Check sheet for the modelled part. Datum: model origin and axes. Units: mm. Face numbers are marked on the shaded views. Coordinates: 2 decimals unless noted, no trailing zeros. Write each loop counter-clockwise with the first axis right and the second up, starting at its lowest first coordinate (ties: lowest second). Pieces come first, ordered by that corner, then holes. Notation, with made-up numbers: (-12, 18.5) - (-5, 18.5) arc R22 cw to (-5, 25.5) - close; hole circle Ø8 at (74.25, 71). An arc over 180 degrees is marked (long way). Use one line per item in the form item = value. Start each with the question number.
1. Draft check along X on the marked faces 1, 2, 3 and 4. Enter one of: +X half, -X half, draft (parallel to the pull), parting line (faces both ways), or undercut.
2. Cross-section at A-A on x = 0. Record the boundary of the cut face in (y, z).
3. Cross-section at C-C on y = 0.75. Record the boundary of the cut face in (x, z).
4. Go/stop test with flat-tipped pins: pin 1 Ø5 at (y, z) = (1, 17) entering from +X; pin 2 Ø2 at (x, y) = (0.5, -1) entering from +Z; pin 3 Ø5.5 at (x, y) = (0, 0) entering from -Z. Record where each tip stops, or that it passes through.
5. Cross-section at B-B on z = -17. Record the boundary of the cut face in (x, y).
6. Scan lines: line 1 along Y through (x, z) = (0, 26.5); line 2 along X through (y, z) = (0, 29.25); line 3 along X through (y, z) = (0, 23.35). Record each from-to range of solid material in increasing order.
7. Cross-section at D-D on y = -5.25. Record the boundary of the cut face in (x, z).
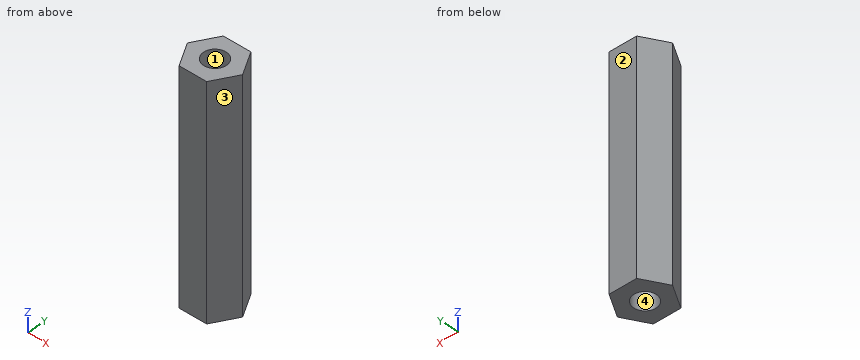
Autodesk Inventor part; units mm, degrees
ref_plane "YZ Plane" through (0, 0, 0) normal (1, 0, 0) x (0, 1, 0)
ref_plane "XZ Plane" through (0, 0, 0) normal (0, 1, 0) x (-1, 0, 0)
ref_plane "XY Plane" through (0, 0, 0) normal (0, 0, 1) x (1, 0, 0)
sketch "Sketch1" plane through (0, 0, 0) normal (0, 0, 1) x (1, 0, 0)
  line L0 (3.6662, 6.35) -> (7.3323, 0)
  line L1 (7.3323, 0) -> (3.6662, -6.35)
  line L2 (3.6662, -6.35) -> (-3.6662, -6.35)
  line L3 (-3.6662, -6.35) -> (-7.3323, 0)
  line L4 (-7.3323, 0) -> (-3.6662, 6.35)
  line L5 (-3.6662, 6.35) -> (3.6662, 6.35)
  circle A0 centre (0, 0) radius 2.0193
  dimension "d0" = 12.7
  dimension "d3" = 4.0386
extrude "Extrusion2" add sketch "Sketch1" along normal mid plane 60.325
sketch "Sketch2" plane through (0, 0, 30.1625) normal (0, 0, 1) x (1, 0, 0)
  point P0 (0, 0)
  point P1 (0, 0)
hole "Hole1" at (0, 0, 30.1625) direction (0, 0, -1) diameter 5.842 depth 7.874 counterbore diameter 6.096 counterbore depth 6.1239
sketch "Sketch3" plane through (0, 0, -30.1625) normal (0, 0, -1) x (-1, 0, 0)
  circle A0 centre (0, 0) radius 2.0193
hole "Hole2" at (0, 0, -30.1625) direction (0, 0, 1) diameter 5.842 depth 7.874 counterbore diameter 6.096 counterbore depth 6.1239
properties part number "1_2 x 2_375-inchHexShaft"
Final values:
q1.face_1 = undercut
q1.face_2 = draft
q1.face_3 = +X half
q1.face_4 = undercut
q2.outline = (-6.35, -30.16) - (-3.05, -30.16) - (-3.05, -24.04) - (-2.92, -24.04) - (-2.92, -22.29) - (-2.02, -22.29) - (-2.02, 22.29) - (-2.92, 22.29) - (-2.92, 24.04) - (-3.05, 24.04) - (-3.05, 30.16) - (-6.35, 30.16) - close; (2.02, -22.29) - (2.92, -22.29) - (2.92, -24.04) - (3.05, -24.04) - (3.05, -30.16) - (6.35, -30.16) - (6.35, 30.16) - (3.05, 30.16) - (3.05, 24.04) - (2.92, 24.04) - (2.92, 22.29) - (2.02, 22.29) - close
q3.outline = (-6.9, -30.16) - (-2.95, -30.16) - (-2.95, -24.04) - (-2.82, -24.04) - (-2.82, -22.29) - (-1.87, -22.29) - (-1.87, 22.29) - (-2.82, 22.29) - (-2.82, 24.04) - (-2.95, 24.04) - (-2.95, 30.16) - (-6.9, 30.16) - close; (1.87, -22.29) - (2.82, -22.29) - (2.82, -24.04) - (2.95, -24.04) - (2.95, -30.16) - (6.9, -30.16) - (6.9, 30.16) - (2.95, 30.16) - (2.95, 24.04) - (2.82, 24.04) - (2.82, 22.29) - (1.87, 22.29) - close
q4.pin_1 = 7.33
q4.pin_2 = 22.29
q4.pin_3 = -22.29
q5.outline = (-7.33, 0) - (-3.67, -6.35) - (3.67, -6.35) - (7.33, 0) - (3.67, 6.35) - (-3.67, 6.35) - close; hole circle Ø4.04 at (0, 0)
q6.line_1 = -6.35 to -3.05, 3.05 to 6.35
q6.line_2 = -7.33 to -3.05, 3.05 to 7.33
q6.line_3 = -7.33 to -2.92, 2.92 to 7.33
q7.outline = (-4.3, -30.16) - (4.3, -30.16) - (4.3, 30.16) - (-4.3, 30.16) - close
